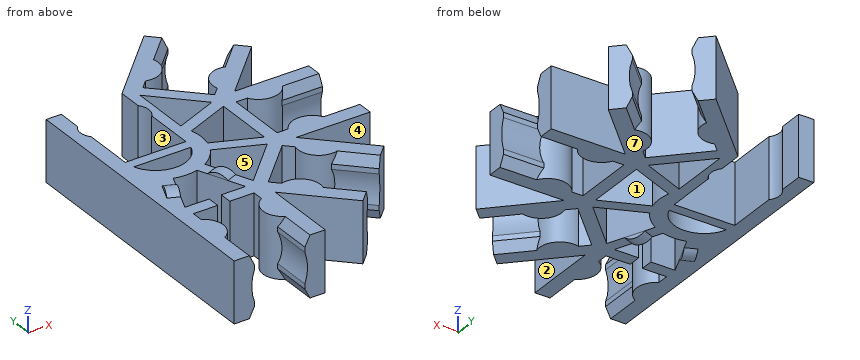
```python
from build123d import *

# Parameters (mm, degrees)
EXTRUDE_1_DEPTH          = 6
EXTRUDE_START            = -3.991967
EXTRUDE_2_DEPTH          = 3.991967
PATTERN_CIRCULAR_1_COUNT = 5
PATTERN_CIRCULAR_1_ANGLE = 180
CUT_EXTRUDE_1_DEPTH      = 7.0000001
EXTRUDE_3_DEPTH          = 1.153683
EXTRUDE_4_DEPTH          = 1.15


with BuildPart() as part:
    # 草图1 → 凸台-拉伸1 (new body)
    with BuildSketch(Plane.XY):
        with BuildLine():
            Line((-4.5, 0), (-4.5, -18.2))
            Line((-4.5, -18.2), (-3, -18.2))
            Line((-3, -18.2), (-3, -14.6))
            ThreePointArc((-3, -14.6), (-1.968245837, -12.85), (-3, -11.1))
            Line((-3, -11.1), (-3, -10))
            Line((-3, -10), (3, -10))
            Line((3, -10), (3, -11.1))
            ThreePointArc((3, -11.1), (1.968245837, -12.85), (3, -14.6))
            Line((3, -14.6), (3, -18.2))
            Line((3, -18.2), (4.5, -18.2))
            Line((4.5, -18.2), (4.5, 0))
            ThreePointArc((4.5, 0), (0, 4.5), (-4.5, 0))
        make_face()
    extrude_1 = extrude(amount=EXTRUDE_1_DEPTH)

    # 草图3 → 凸台-拉伸2 (add)
    with BuildSketch(Plane.XZ.offset(18.2).offset(EXTRUDE_START)):
        with BuildLine():
            Line((-3, 6), (-3, 0))
            Line((-3, 0), (-2.5, 1))
            Line((-2.5, 1), (-2.5, 1.5))
            ThreePointArc((-2.5, 1.5), (-2.757359313, 3), (-2.5, 4.5))
            Line((-2.5, 4.5), (-2.5, 5))
            Line((-2.5, 5), (-3, 6))
        make_face()
        with BuildLine():
            Line((3, 0), (2.5, 1))
            Line((2.5, 1), (2.5, 1.5))
            ThreePointArc((2.5, 1.5), (2.757359313, 3), (2.5, 4.5))
            Line((2.5, 4.5), (2.5, 5))
            Line((2.5, 5), (3, 6))
            Line((3, 6), (3, 0))
        make_face()
    extrude_2 = extrude(amount=EXTRUDE_2_DEPTH)

    # 阵列(圆周)1: 凸台-拉伸1, 凸台-拉伸2 ×5 about axis
    pattern_circular_1_axis = Axis((0, 0, 0), (0, 0, 1))
    for i in range(1, PATTERN_CIRCULAR_1_COUNT):
        add(extrude_1.rotate(pattern_circular_1_axis, i * PATTERN_CIRCULAR_1_ANGLE / (PATTERN_CIRCULAR_1_COUNT - 1)))
        add(extrude_2.rotate(pattern_circular_1_axis, i * PATTERN_CIRCULAR_1_ANGLE / (PATTERN_CIRCULAR_1_COUNT - 1)))

    # 草图4 → 切除-拉伸1 (cut, through all)
    with BuildSketch(Plane(origin=(0, 0, 0), x_dir=(-1, 0, 0), z_dir=(0, 0, -1))):
        with BuildLine():
            Line((-3, -8.75), (-1.174936357, -4.343906601))
            ThreePointArc((-1.174936357, -4.343906601), (0, -4.5), (1.174936357, -4.343906601))
            Line((1.174936357, -4.343906601), (3, -8.75))
            Line((3, -8.75), (0.6, -8.75))
            Line((0.6, -8.75), (0.6, -10))
            Line((0.6, -10), (-0.6, -10))
            Line((-0.6, -10), (-0.6, -8.75))
            Line((-0.6, -8.75), (-3, -8.75))
        make_face()
        with BuildLine():
            Line((-4.065863992, -8.308504679), (-8.308504679, -4.065863992))
            Line((-8.308504679, -4.065863992), (-3.90241128, -2.240800349))
            ThreePointArc((-3.90241128, -2.240800349), (-3.181980515, -3.181980515), (-2.240800349, -3.90241128))
            Line((-2.240800349, -3.90241128), (-4.065863992, -8.308504679))
        make_face()
        with BuildLine():
            Line((-8.75, 3), (-4.343906601, 1.174936357))
            ThreePointArc((-4.343906601, 1.174936357), (-4.5, 0), (-4.343906601, -1.174936357))
            Line((-4.343906601, -1.174936357), (-8.75, -3))
            Line((-8.75, -3), (-8.75, 3))
        make_face()
        Polygon((-8.308504679, 4.065863992), (-4.065863992, 2.308504679), (-4.065863992, 8.308504679), align=None)
        with BuildLine():
            Line((-4.5, 10.863961031), (-3, 9.363961031))
            Line((-3, 9.363961031), (-3, 7))
            ThreePointArc((-3, 7), (-3.381966011, 6), (-3, 5))
            Line((-3, 5), (-3, 0))
            Line((-3, 0), (0, 0))
            Line((0, 0), (3, 0))
            Line((3, 0), (3, 5))
            ThreePointArc((3, 5), (3.381966011, 6), (3, 7))
            Line((3, 7), (3, 9.363961031))
            Line((3, 9.363961031), (4.5, 9.363961031))
            Line((4.5, 9.363961031), (4.5, 18.2))
            Line((4.5, 18.2), (-4.5, 18.2))
            Line((-4.5, 18.2), (-4.5, 10.863961031))
        make_face()
        with BuildLine():
            Line((-2.828427125, -1), (2.828427125, -1))
            ThreePointArc((2.828427125, -1), (0, -3), (-2.828427125, -1))
        make_face()
    extrude(amount=-CUT_EXTRUDE_1_DEPTH, mode=Mode.SUBTRACT)

    # 草图5 → 凸台-拉伸3 (add)
    with BuildSketch(Plane(origin=(-0.532931996, -0.220747661, 0), x_dir=(0, 0, 1), z_dir=(-0.923879533, -0.382683432, 0))):
        with BuildLine():
            Line((0, -7.5), (0, -5.5))
            ThreePointArc((0, -5.5), (-0.381966011, -6.5), (0, -7.5))
        make_face()
        with BuildLine():
            Line((6, -7.5), (6, -5.5))
            ThreePointArc((6, -5.5), (6.381966011, -6.5), (6, -7.5))
        make_face()
    extrude(amount=-EXTRUDE_3_DEPTH)

    # 草图7 → 凸台-拉伸4 (add)
    with BuildSketch(Plane(origin=(0.532931996, -0.220747661, 0), x_dir=(0, 0, -1), z_dir=(0.923879533, -0.382683432, 0))):
        with BuildLine():
            Line((0, -7.5), (0, -5.5))
            ThreePointArc((0, -5.5), (0.381966011, -6.5), (0, -7.5))
        make_face()
        with BuildLine():
            Line((-6, -7.5), (-6, -5.5))
            ThreePointArc((-6, -5.5), (-6.381966011, -6.5), (-6, -7.5))
        make_face()
    extrude(amount=-EXTRUDE_4_DEPTH)


solid = part.part
```
Here's how the part is built. I have some questions about the finished solid (model axes, mm). Face numbers are marked on the shaded views. A direction names the side the tool comes from. Give positions to 0.01 mm unless a question says otherwise; leave off trailing zeros. Loops run counter-clockwise (first coordinate to the right, second up) from the corner with the lowest first, then second, coordinate; pieces in that order, holes last. Notation, with made-up numbers: M 18.5,-3.5 L 42.5,-3.5 A25 ccw 42.5,33.5 Z; hole C 18,-30.5 d1. An arc over 180 degrees is marked long. Put each result on its own line as item: value. Start each with the question number.
(1) I want a section at B-B on y = 7.5. Please give me the cut outline in (x, z), then the cut area to 3 significant figures.
(2) I want a section at A-A on x = 6.25. Please give me the cut outline in (y, z).
(3) If we mould it in two halves opening along Z, with no side actions, what happens to the marked faces 5, 6 and 7? For each: +Z half, -Z half, draft (parallel to the pull), parting line (faces both ways), or undercut.
(4) I want a section at C-C on z = 3. State how many separate pieces and enclosed holes the cut face has, then the cut area to 3 significant figures.
(5) I need wall thicknesses on line 1 along X through (y, z) = (-7.5, 4.5); line 2 along X through (y, z) = (-12.5, 5.25); line 3 along X through (y, z) = (-2.5, 5.5). Which ranges of each line are inside material? Lowest first, please. Write a range as [from, to].
(6) Will these pins go through, and if not, where does the flat tip stop? pin 1 Ø2.5 at (y, z) = (7.5, 2) entering from +X; pin 2 Ø3 at (y, z) = (-8, 1) entering from +X; pin 3 Ø0.5 at (x, z) = (10.5, 2) entering from -Y; pin 4 Ø2.5 at (x, z) = (-2.5, 2) entering from -Y.
(7) For the marked faces 1, 2, 3 and 4, which set-ups out of +Z, -Z, +X, -X, +Y, -Y let a thin tool reach every point of the face, with its end or its side?
Answer block:
1. outline: M -4.5,0 L -3,0 L -3,6 L -4.5,6 Z; M 3,0 L 4.07,0 L 4.07,6 L 3,6 Z; M 4.87,0 L 6.64,0 L 6.64,6 L 4.87,6 Z; M 10.31,0 L 13.86,0 L 13.86,6 L 10.31,6 Z
1. area: 47.3 mm^2
2. outline: M -12.61,0 L -9.89,0 L -9.89,6 L -12.61,6 Z; M -7.89,0 L -6.12,0 L -6.12,6 L -7.89,6 Z; M -3.21,0 L -1.96,0 L -1.96,6 L -3.21,6 Z; M 1.96,0 L 3.21,0 L 3.21,6 L 1.96,6 Z; M 6.12,0 L 7.89,0 L 7.89,6 L 6.12,6 Z; M 9.89,0 L 12.61,0 L 12.61,6 L 9.89,6 Z
3. face 5: draft
3. face 6: undercut
3. face 7: -Z half
4. separate pieces: 1
4. enclosed holes: 4
4. area: 242 mm^2
5. line 1: [-4.5, -2.48], [2.48, 3.73], [4.87, 6.64], [10.31, 13.86]
5. line 2: [-4.5, -2], [2, 4.5], [6.14, 8.79]
5. line 3: [-4.5, -1.66], [1.66, 3.74], [4.53, 7.54], [8.75, 10], [11.49, 14.21]
6. pin 1: x = 15.11
6. pin 2: x = 15.86
6. pin 3: y = -15.49
6. pin 4: y = -18.2
7. face 1: +Z, -Z
7. face 2: +Z, -Z, -Y
7. face 3: +Z, -Z, +Y
7. face 4: +Z, -Z, +X
